```python
from build123d import *

# Parameters (mm, degrees)
SKETCH_1_W      = 150
SKETCH_1_H      = 85
SKETCH_1_R      = 2.25
SKETCH_1_R_2    = 1.75
EXTRUDE_1_DEPTH = 1.5


with BuildPart() as part:
    # Эскиз1 → Вытянуть1 (new body)
    with BuildSketch(Plane.XY):
        Rectangle(SKETCH_1_W, SKETCH_1_H)
        with Locations((-70, 37.5)):
            Circle(SKETCH_1_R, mode=Mode.SUBTRACT)
        with Locations(Location((-70, -37.5, 0), (0, 0, 180))):
            Circle(SKETCH_1_R, mode=Mode.SUBTRACT)
        with Locations((70, -37.5)):
            Circle(SKETCH_1_R, mode=Mode.SUBTRACT)
        with Locations(Location((70, 37.5, 0), (0, 0, 180))):
            Circle(SKETCH_1_R, mode=Mode.SUBTRACT)
        with Locations((-50, 32.5)):
            Circle(SKETCH_1_R_2, mode=Mode.SUBTRACT)
        with Locations(Location((-50, -37.5, 0), (0, 0, 180))):
            Circle(SKETCH_1_R_2, mode=Mode.SUBTRACT)
        with Locations((50, 32.5)):
            Circle(SKETCH_1_R_2, mode=Mode.SUBTRACT)
        with Locations(Location((50, -37.5, 0), (0, 0, 180))):
            Circle(SKETCH_1_R_2, mode=Mode.SUBTRACT)
    extrude(amount=EXTRUDE_1_DEPTH)


solid = part.part
```
Can you work these out from the model? Positions are in its coordinate system, mm. Give positions to 0.01 mm unless a question says otherwise; leave off trailing zeros. Loops run counter-clockwise (first coordinate to the right, second up) from the corner with the lowest first, then second, coordinate; pieces in that order, holes last. Notation, with made-up numbers: M -19.75,-12.5 L 36.25,-12.5 A8 ccw 36.25,-6.5 Z; hole C -0.75,23 d11. An arc over 180 degrees is marked long. Use one line per item in the form item = value. Start each with the question number.
(1) I want a section at B-B, the plane x = 70. Write out the boundary of the cut face in (y, z).
(2) I want a section at A-A, the plane y = 37.5. Write out the boundary of the cut face in (x, z), and give its area (4 significant figures).
(3) Thinking about a two-plate mould opening in Y: for faces 1 (the flat face through (-1, 1, 0)), 2 (the cylindrical face through (-68.79, 39.397, 0.74)), which applies, released by +Y, released by -Y, zero draft, split by the parting line, or undercut?
(4) I want a section at C-C, the plane y = -37.5. Write out the boundary of the cut face in (x, z).
(5) I'm going to push a flat-ended pin straight in: P1, Ø2, axis at x = -50, y = 32.5, coming from the -Z side. Where does the tip first touch, or does it pass through?
(6) Please list where these lines run through material, in increasing order: line 1 (Y direction, x = 70, z = 0.7); line 2 (Y direction, x = 50, z = 0.5).
Worked out:
q1.outline = M -42.5,0 L -39.75,0 L -39.75,1.5 L -42.5,1.5 Z; M -35.25,0 L 35.25,0 L 35.25,1.5 L -35.25,1.5 Z; M 39.75,0 L 42.5,0 L 42.5,1.5 L 39.75,1.5 Z
q2.outline = M -75,0 L -72.25,0 L -72.25,1.5 L -75,1.5 Z; M -67.75,0 L 67.75,0 L 67.75,1.5 L -67.75,1.5 Z; M 72.25,0 L 75,0 L 75,1.5 L 72.25,1.5 Z
q2.area = 211.5 mm²
q3.face_1 = zero draft
q3.face_2 = undercut
q4.outline = M -75,0 L -72.25,0 L -72.25,1.5 L -75,1.5 Z; M -67.75,0 L -51.75,0 L -51.75,1.5 L -67.75,1.5 Z; M -48.25,0 L 48.25,0 L 48.25,1.5 L -48.25,1.5 Z; M 51.75,0 L 67.75,0 L 67.75,1.5 L 51.75,1.5 Z; M 72.25,0 L 75,0 L 75,1.5 L 72.25,1.5 Z
q5.P1 = through
q6.line_1 = -42.5 to -39.75, -35.25 to 35.25, 39.75 to 42.5
q6.line_2 = -42.5 to -39.25, -35.75 to 30.75, 34.25 to 42.5
